Check sheet for the drawn part. Datum: minimum x, y, z corner. Units: mm. A direction names the side the tool comes from. Round coordinates to 2 decimals unless told otherwise and drop trailing zeros. Order: outer loops, then holes, each group sorted by start corner. A loop starts at its lowest first (then second) coordinate and runs counter-clockwise, first axis right, second up. Notation, with made-up numbers: M 22,5 L 68,5 A22 ccw 68,31 Z; hole C -36,-22 d8. An arc over 180 degrees is marked long. Use one line per item in the form item = value. Start each with the question number.
Item 1: Cross-section at B-B on z = 5.5. Enter the section's corners in (x, y).
Item 2: Cross-section at A-A on y = 6.5. Enter the section's corners in (x, z), then the cut area to 3 significant figures.
Item 3: Go/stop test with flat-tipped pins: pin 1 Ø6 at (x, y) = (16.5, 11.5) entering from +Z; pin 2 Ø3 at (x, y) = (19.5, 24) entering from +Z. Record where each tip stops, or that it passes through.
Item 4: Cross-section at C-C on x = 19. Enter the section's corners in (y, z), then the cut area to 3 significant figures.
Item 5: Tool access check on the marked faces 5, 6 and 7. Record the directions out of +Z, -Z, +X, -X, +Y, -Y that give a thin tool (end or side, any length) a straight path to the whole face; none if there is none.
Item 6: Release check for a two-part mould opening along X. For the marked faces 1, 2, 3 and 4 record: +X half, -X half, draft (parallel to the pull), parting line (faces both ways), or undercut.
Item 7: Thickness scan on probe 1 along X at (y, z) = (9.25, 7); probe 2 along Z at (x, y) = (21.5, 6); probe 3 along Y at (x, z) = (16, 7.25). Record the ranges inside material, lowest first. Write a range as [from, to].
Item 8: Cross-section at D-D on y = 26. Enter the section's corners in (x, z).
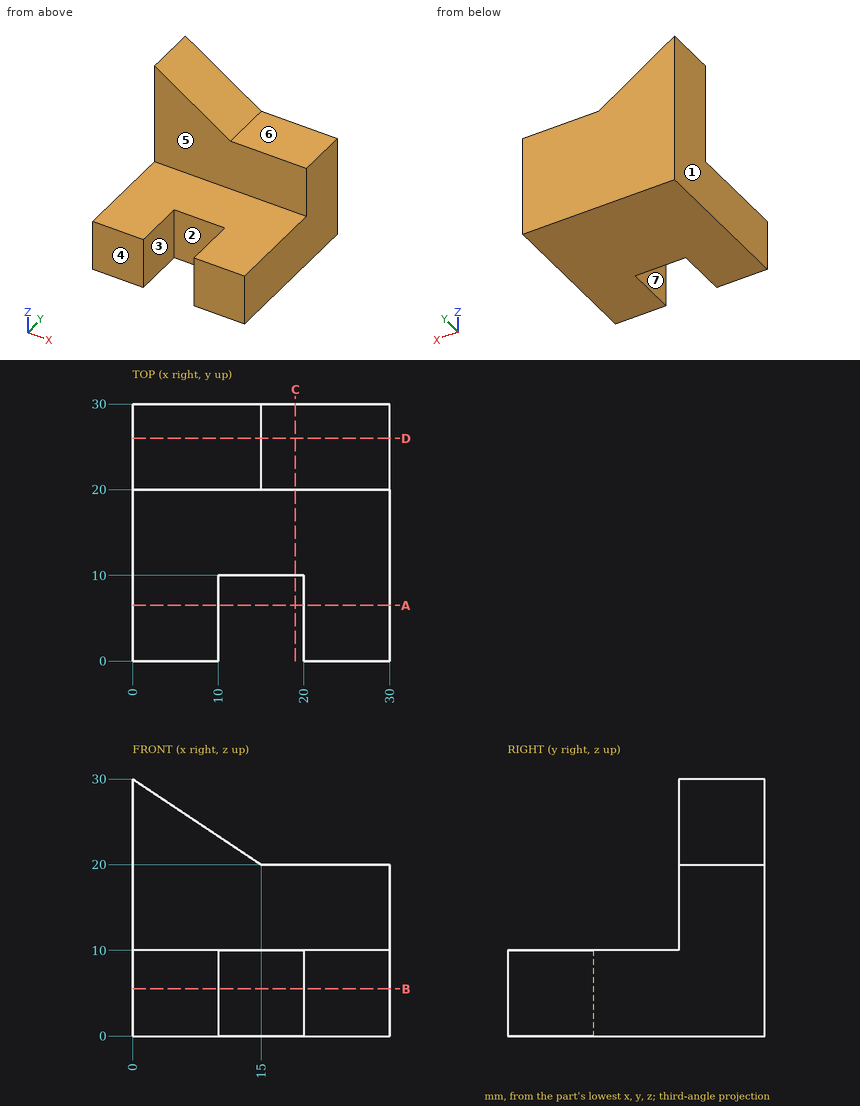
Output values:
q1.outline = M 0,0 L 10,0 L 10,10 L 20,10 L 20,0 L 30,0 L 30,30 L 0,30 Z
q2.outline = M 0,0 L 10,0 L 10,10 L 0,10 Z; M 20,0 L 30,0 L 30,10 L 20,10 Z
q2.area = 200 mm2
q3.pin_1 = 10
q3.pin_2 = 20
q4.outline = M 10,0 L 30,0 L 30,20 L 20,20 L 20,10 L 10,10 Z
q4.area = 300 mm2
q5.face_5 = +Z, +X, -X, -Y
q5.face_6 = +Z, +X, +Y, -Y
q5.face_7 = +Z, -Z, -Y
q6.face_1 = -X half
q6.face_2 = undercut
q6.face_3 = undercut
q6.face_4 = draft
q7.probe_1 = [0, 10], [20, 30]
q7.probe_2 = [0, 10]
q7.probe_3 = [10, 30]
q8.outline = M 0,0 L 30,0 L 30,20 L 15,20 L 0,30 Z
